Job drawing, mm, ordinate dimensions from the low corner. One solid piece. Round coordinates to 2 decimals unless told otherwise and drop trailing zeros. Loops run counter-clockwise (first coordinate to the right, second up) from the corner with the lowest first, then second, coordinate; pieces in that order, holes last.
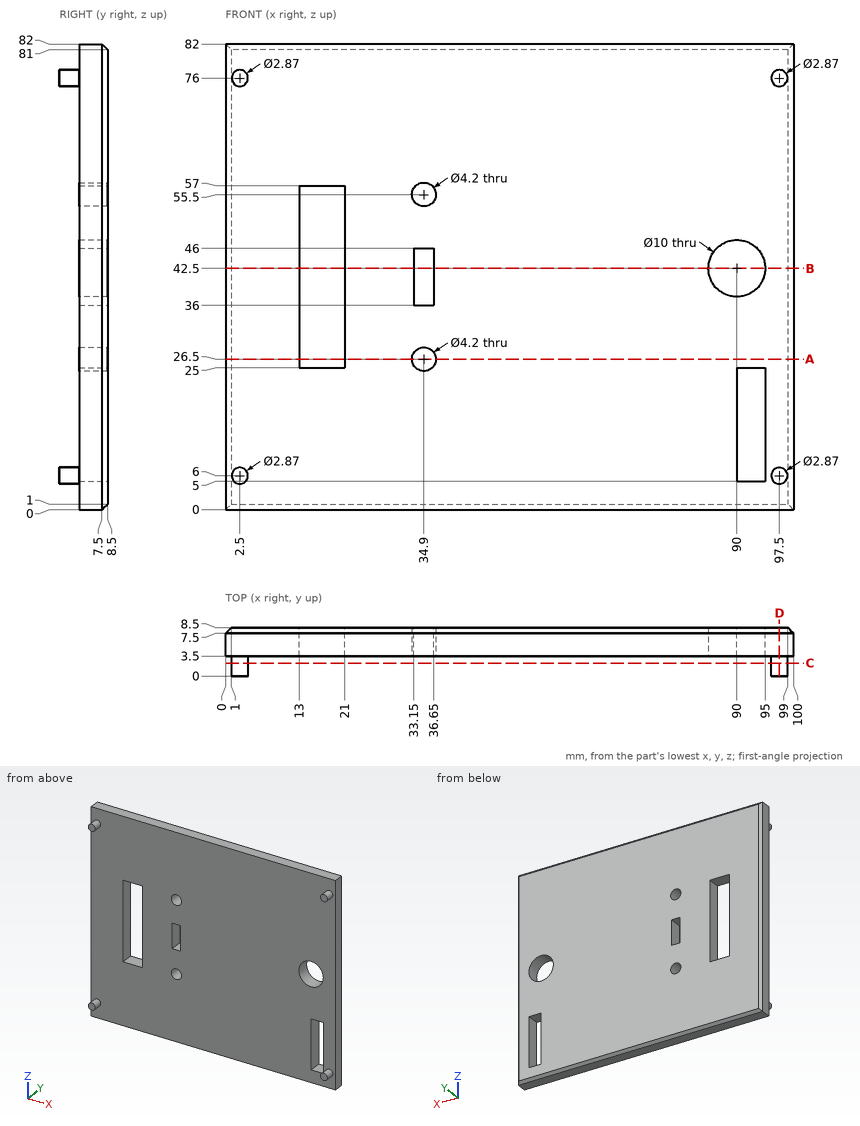
1) Slice it at A-A, the plane z = 26.5. Give the cut face in (x, y), then the cut area to 3 significant figures.
Values:
outline: (0, 3.5) - (13, 3.5) - (13, 8.5) - (1, 8.5) - (0, 7.5) - close; (21, 3.5) - (32.8, 3.5) - (32.8, 8.5) - (21, 8.5) - close; (37, 3.5) - (100, 3.5) - (100, 7.5) - (99, 8.5) - (37, 8.5) - close
area: 438 mm2
2) Slice it at C-C, the plane y = 2.25. Give the cut face in (x, z) (3 decimals).
Values:
outline: circle Ø2.87 at (2.5, 6); circle Ø2.87 at (2.5, 76); circle Ø2.87 at (97.5, 6); circle Ø2.87 at (97.5, 76)
3) Slice it at D-D, the plane x = 97.5. Give the cut face in (y, z) (3 decimals).
Values:
outline: (0, 4.565) - (3.5, 4.565) - (3.5, 0) - (7.5, 0) - (8.5, 1) - (8.5, 81) - (7.5, 82) - (3.5, 82) - (3.5, 77.435) - (0, 77.435) - (0, 74.565) - (3.5, 74.565) - (3.5, 7.435) - (0, 7.435) - close
4) Drop flat-ended pins along their axis: pin 1 Ø3.5 at (x, z) = (34.9, 26.5) entering from +Y; pin 2 Ø8 at (x, z) = (48, 11) entering from -Y. Give the stop position or say it passes through.
Values:
pin 1: passes through
pin 2: stops at y = 3.5
5) Wall check: line 1 along X through (y, z) = (4.75, 26.5); line 2 along X through (y, z) = (6.55, 42.5); line 3 along X through (y, z) = (6.5, 41). Give the ranges that are in metal, low to high.
Values:
line 1: x = 0 to 13, 21 to 32.8, 37 to 100
line 2: x = 0 to 13, 21 to 33.15, 36.65 to 85, 95 to 100
line 3: x = 0 to 13, 21 to 33.15, 36.65 to 85.23, 94.77 to 100
6) Slice it at B-B, the plane z = 42.5. Give the cut face in (x, y).
Values:
outline: (0, 3.5) - (13, 3.5) - (13, 8.5) - (1, 8.5) - (0, 7.5) - close; (21, 3.5) - (33.15, 3.5) - (33.15, 8.5) - (21, 8.5) - close; (36.65, 3.5) - (85, 3.5) - (85, 8.5) - (36.65, 8.5) - close; (95, 3.5) - (100, 3.5) - (100, 7.5) - (99, 8.5) - (95, 8.5) - close
